```python
from build123d import *

# Parameters (mm, degrees)
F1_DEPTH = 6.5
F2_DEPTH = 30
F3_DEPTH = 2.5
F0_W     = 29.5
F0_H     = 61.4
F4_DEPTH = 2.5
F5_W     = 45.5
F5_H     = 5.322864
F6_DEPTH = 25


with BuildPart() as f1:
    # F0 (on Top) → F1 (new body)
    with BuildSketch(Plane.XY):
        Polygon((-58.032156, 36.652669), (-58.032156, 30.152669), (-64.532156, 30.152669), (-64.532156, 23.652669), (-58.032156, 23.652669), (-58.032156, 17.152669), (-64.532156, 17.152669), (-64.532156, 10.652669), (-58.032156, 10.652669), (-58.032156, 4.152669), (-64.532156, 4.152669), (-64.532156, -2.347331), (-58.032156, -2.347331), (-58.032156, -8.847331), (-64.532156, -8.847331), (-64.532156, -15.347331), (-58.032156, -15.347331), (-58.032156, -21.847331), (-64.532156, -21.847331), (-64.532156, -28.347331), (-58.032156, -28.347331), (-58.032156, -34.847331), (-64.532156, -34.847331), (-64.532156, -41.347331), (-58.032156, -41.347331), (-58.032156, -53.445331), (58.967844, -53.445331), (58.967844, -41.347331), (65.467844, -41.347331), (65.467844, -34.847331), (58.967844, -34.847331), (58.967844, -28.347331), (65.467844, -28.347331), (65.467844, -21.847331), (58.967844, -21.847331), (58.967844, -15.347331), (65.467844, -15.347331), (65.467844, -8.847331), (58.967844, -8.847331), (58.967844, -2.347331), (65.467844, -2.347331), (65.467844, 4.152669), (58.967844, 4.152669), (58.967844, 10.652669), (65.467844, 10.652669), (65.467844, 17.152669), (58.967844, 17.152669), (58.967844, 23.652669), (58.967844, 30.152669), (52.467844, 30.152669), (52.467844, 36.652669), (45.967844, 36.652669), (45.967844, 30.152669), (39.467844, 30.152669), (39.467844, 36.652669), (32.967844, 36.652669), (32.967844, 30.152669), (26.467844, 30.152669), (26.467844, 36.652669), (19.967844, 36.652669), (19.967844, 30.152669), (13.467844, 30.152669), (13.467844, 36.652669), (6.967844, 36.652669), (6.967844, 30.152669), (0.467844, 30.152669), (0.467844, 36.652669), (-6.032156, 36.652669), (-6.032156, 30.152669), (-12.532156, 30.152669), (-12.532156, 36.652669), (-19.032156, 36.652669), (-19.032156, 30.152669), (-25.532156, 30.152669), (-25.532156, 36.652669), (-32.032156, 36.652669), (-32.032156, 30.152669), (-38.532156, 30.152669), (-38.532156, 36.652669), (-45.032156, 36.652669), (-45.032156, 30.152669), (-51.532156, 30.152669), (-51.532156, 36.652669), align=None)
    extrude(amount=F1_DEPTH)


with BuildPart() as f2:
    # F0 (on Top) → F2 (new body)
    with BuildSketch(Plane.XY):
        Polygon((224.515274, 15.340945), (114.015274, 15.340945), (114.015274, 10.340945), (143.515274, 10.340945), (143.515274, -51.059055), (146.515274, -51.059055), (146.515274, 10.018081), (192.015274, 10.018081), (192.015274, -51.059055), (195.015274, -51.059055), (195.015274, 10.340945), (224.515274, 10.340945), align=None)
    extrude(amount=F2_DEPTH)

    # F2_face (on face) → F3 (join)
    with BuildSketch(Plane(origin=(169.265274, -0.273746, 0), x_dir=(1, 0, 0), z_dir=(0, 0, -1))):
        Polygon((55.25, -10.614691), (25.75, -10.614691), (25.75, 50.785309), (22.75, 50.785309), (22.75, -10.291827), (-22.75, -10.291827), (-22.75, 50.785309), (-25.75, 50.785309), (-25.75, -10.614691), (-55.25, -10.614691), (-55.25, -15.614691), (55.25, -15.614691), align=None)
    extrude(amount=F3_DEPTH)

    # F0 (on Top) → F4 (join)
    with BuildSketch(Plane.XY):
        with Locations((209.765274, -20.359055)):
            Rectangle(F0_W, F0_H)
        with Locations((128.765274, -20.359055)):
            Rectangle(F0_W, F0_H)
    extrude(amount=-F4_DEPTH)

    # F5 (on face) → F6 (cut)
    with BuildSketch(Plane(origin=(0, 0, -2.5), x_dir=(1, 0, 0), z_dir=(0, 0, -1))):
        with Locations((169.265274, -12.679513)):
            Rectangle(F5_W, F5_H)
    extrude(amount=-F6_DEPTH, mode=Mode.SUBTRACT)


with BuildPart() as f7_1:
    # F7: copy of F2
    add(f2.part)


solid = f7_1.part
```
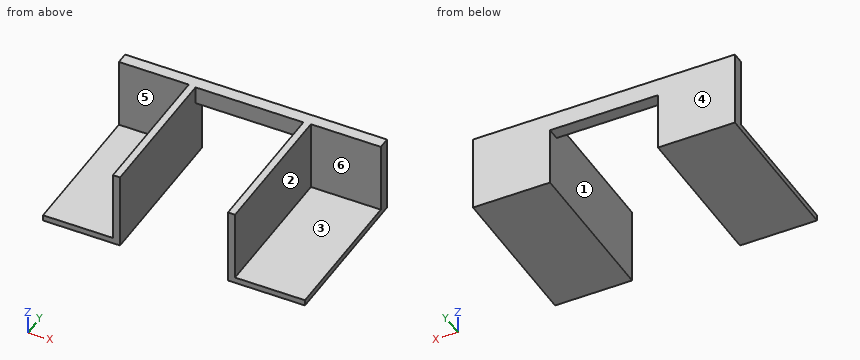
Design review of the part built by this model. Coordinates are the model's own, in mm. Face numbers are marked on the shaded views. A direction names the side the tool comes from. Coordinates: 2 decimals unless noted, no trailing zeros. Order: outer loops, then holes, each group sorted by start corner. A loop starts at its lowest first (then second) coordinate and runs counter-clockwise, first axis right, second up. Notation, with made-up numbers: (-36, -20) - (-19, -20) arc R28 cw to (-19, 5) - close; hole circle Ø10 at (41, -32.5). An arc over 180 degrees is marked (long way). One line per question, with ' | ' between items.
Q1. Consider section C-C, the plane x = 202.5. Give the boundary of the cut face in (y, z).
Answer key:
outline: (-51.06, -2.5) - (15.34, -2.5) - (15.34, 30) - (10.34, 30) - (10.34, 0) - (-51.06, 0) - close
Q2. For the marked faces 4, 5 and 6, list the 3-axis set-ups (+Z, -Z, +X, -X, +Y, -Y) from which the entire face can be reached by the end or side of a thin tool; tool diameter is ignored.
Answer key:
face 4: +Z, -Z, +X, -X, +Y | face 5: +Z, -X, -Y | face 6: +Z, +X, -Y
Q3. The part is to be moulded in two halves that separate along X. For the marked faces 1, 2 and 3, say which applies: +X half, -X half, draft (parallel to the pull), parting line (faces both ways), or undercut.
Answer key:
face 1: undercut | face 2: +X half | face 3: draft
Q4. To check wall thickness, follow line 1 along X through (y, z) = (-27, 19.5); line 2 along X through (y, z) = (12.5, -0.5); line 3 along Z through (x, y) = (204.5, -39). State the ranges of each line that lie inside material, in increasing order.
Answer key:
line 1: x = 143.52 to 146.52, 192.02 to 195.02 | line 2: x = 114.02 to 146.52, 192.02 to 224.52 | line 3: z = -2.5 to 0
Q5. Clearance check with flat-ended pins moving along their axes: pin 1 Ø15 at (x, z) = (128, 14) entering from -Y; pin 2 Ø15 at (y, z) = (-11.5, 8) entering from +X; pin 3 Ø2 at (x, y) = (128, -9.5) entering from +Z. State where each tip first meets the part, or that it passes through.
Answer key:
pin 1: stops at y = 10.34 | pin 2: stops at x = 195.02 | pin 3: stops at z = 0
Q6. Consider section A-A, the plane y = -16. Give the boundary of the cut face in (x, z), then the cut area to 4 significant figures.
Answer key:
outline: (114.02, -2.5) - (146.52, -2.5) - (146.52, 30) - (143.52, 30) - (143.52, 0) - (114.02, 0) - close; (192.02, -2.5) - (224.52, -2.5) - (224.52, 0) - (195.02, 0) - (195.02, 30) - (192.02, 30) - close | area: 342.5 mm2
Q7. Consider section D-D, the plane x = 174.5. Give the boundary of the cut face in (y, z), then the cut area to 3 significant figures.
Answer key:
outline: (10.02, 22.5) - (15.34, 22.5) - (15.34, 30) - (10.02, 30) - close | area: 39.9 mm2
Q8. Consider section B-B, the plane z = 2. Give the boundary of the cut face in (x, y), then the cut area to 3 significant figures.
Answer key:
outline: (114.02, 10.34) - (143.52, 10.34) - (143.52, -51.06) - (146.52, -51.06) - (146.52, 15.34) - (114.02, 15.34) - close; (192.02, -51.06) - (195.02, -51.06) - (195.02, 10.34) - (224.52, 10.34) - (224.52, 15.34) - (192.02, 15.34) - close | area: 693 mm2
